Source: CAD feature listing. Evaluate the final solid. Frame: model axes, mm. Face numbers are marked on the shaded views. A direction names the side the tool comes from. Round coordinates to 2 decimals unless told otherwise and drop trailing zeros. Answer in a Markdown table with one row per item. Add a question column.
Item 1: Contact query for flat-ended pins moving along their axis: pin 1 (12 mm diameter, centred on x = 77.5, y = -34, fed in from -Z); pin 2 (5 mm diameter, centred on x = 42, y = -41.5, fed in from +Z); pin 3 (5 mm diameter, centred on x = 20, y = 10, fed in from +Z). Output: stop coordinate, or through.
Item 2: Set-up query: the marked faces 1 and 2. Return all of +Z, -Z, +X, -X, +Y, -Y with unobstructed straight access to the full face (end or side cutting, diameter ignored); none if empty.
Item 3: Material intervals for probe 1 along X at (y, z) = (31, 40); probe 2 along Z at (x, y) = (73, -0.5); probe 3 along Z at (x, y) = (87, 34), sorted ascending.
from build123d import *

# Parameters (mm, degrees)
SKETCH6_R           = 44.45
BOSS_EXTRUDE3_DEPTH = 10


with BuildPart() as part:
    # Sketch1 for Loft3 → Loft3 section 0
    with BuildSketch(Plane(origin=(0, 0, 0), x_dir=(0, 0, 1), z_dir=(1, 0, 0))):
        with BuildLine():
            Line((-35, -54.5), (35, -54.5))
            # circular arc as an exact rational Bezier (weights 1, cos(half-angle), 1)
            Bezier((35, -54.5), (67.45879246, 0), (35, 54.5), weights=[1, 0.859165949, 1])
            Line((35, 54.5), (-35, 54.5))
            Bezier((-35, 54.5), (-67.45879246, 0), (-35, -54.5), weights=[1, 0.859165949, 1])
        make_face()
    # Sketch5 for Loft3 → Loft3 section 1
    with BuildSketch(Plane(origin=(148, 148, 0), x_dir=(0, -1, 0), z_dir=(1, 0, 0))):
        with BuildLine():
            Line((93.5, 35), (93.5, -35))
            Bezier((93.5, -35), (148, -67.45879246), (202.5, -35), weights=[1, 0.859165949, 1])
            Line((202.5, -35), (202.5, 35))
            Bezier((202.5, 35), (148, 67.45879246), (93.5, 35), weights=[1, 0.859165949, 1])
        make_face()
    loft()

    # Sketch6 → Boss-Extrude3 (add)
    with BuildSketch(Plane(origin=(148, 0, 0), x_dir=(0, 0, -1), z_dir=(1, 0, 0))):
        Circle(SKETCH6_R)
    extrude(amount=BOSS_EXTRUDE3_DEPTH)


solid = part.part
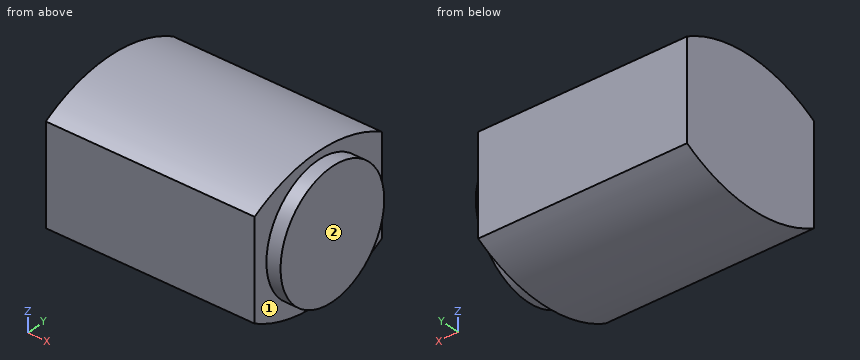
Results below:
| question | item | result |
|---|---|---|
| 1 | pin 1 | z = -46.25 |
| 1 | pin 2 | z = 42.6 |
| 1 | pin 3 | z = 49.74 |
| 2 | face 1 | +X |
| 2 | face 2 | +Z, -Z, +X, +Y, -Y |
| 3 | probe 1 | 0 to 148 |
| 3 | probe 2 | -50 to 50 |
| 3 | probe 3 | -44.43 to 44.43 |
